Geometry check sheet. Reference: the model listing, model coordinates, mm. Face numbers are marked on the shaded views. A direction names the side the tool comes from. Coordinates: 2 decimals unless noted, no trailing zeros. Loops run counter-clockwise (first coordinate to the right, second up) from the corner with the lowest first, then second, coordinate; pieces in that order, holes last. Notation, with made-up numbers: (-7.5, -34.5) - (49.5, -34.5) arc R23 ccw to (49.5, -16.5) - close; hole circle Ø8 at (-13, 4.5). An arc over 180 degrees is marked (long way). One line per item, written item: value.
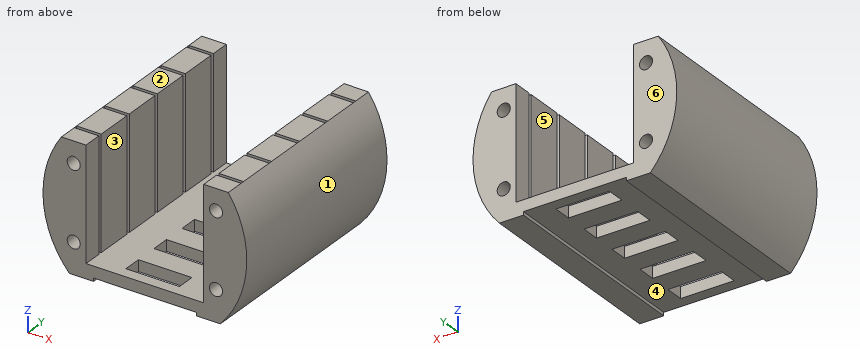
from build123d import *

# Parameters (mm, degrees)
BOSS_EXTRUDE2_DEPTH = 100
SKETCH2_W           = 26
SKETCH2_H           = 9
CUT_EXTRUDE1_DEPTH  = 10
SKETCH3_W           = 81.1
SKETCH3_H           = 1.7
CUT_EXTRUDE2_DEPTH  = 54.585490237
LPATTERN1_COUNT     = 5
LPATTERN1_PITCH     = 20
CUT_EXTRUDE3_START  = -100
SKETCH5_R           = 3.175
CUT_EXTRUDE3_DEPTH  = 100


with BuildPart() as part:
    # Sketch1 → Boss-Extrude2 (new body)
    with BuildSketch(Plane(origin=(0, 0, 0), x_dir=(1, 0, 0), z_dir=(0, 1, 0))):
        with BuildLine():
            Line((-40.55, -28.441490819), (-28.616848255, -28.441490819))
            Line((-28.616848255, -28.441490819), (-28.616848255, 26.143999418))
            Line((-28.616848255, 26.143999418), (28.616848255, 26.143999418))
            Line((28.616848255, 26.143999418), (28.616848255, -28.441490819))
            Line((28.616848255, -28.441490819), (40.55, -28.441490819))
            ThreePointArc((40.55, -28.441490819), (49.434601237, 3.072637396), (36.715901224, 33.243999418))
            Line((36.715901224, 33.243999418), (25, 33.243999418))
            Line((25, 33.243999418), (25, 31.643999418))
            Line((25, 31.643999418), (-25, 31.643999418))
            Line((-25, 31.643999418), (-25, 33.243999418))
            Line((-25, 33.243999418), (-36.715901224, 33.243999418))
            ThreePointArc((-36.715901224, 33.243999418), (-49.434601237, 3.072637396), (-40.55, -28.441490819))
        make_face()
    extrude(amount=BOSS_EXTRUDE2_DEPTH)

    # Sketch2 → Cut-Extrude1 (cut)
    with BuildSketch(Plane.XY.offset(-26.143999418)):
        with Locations((0, 10)):
            Rectangle(SKETCH2_W, SKETCH2_H)
    cut_extrude1 = extrude(amount=-CUT_EXTRUDE1_DEPTH, mode=Mode.SUBTRACT)

    # Sketch3 → Cut-Extrude2 (cut)
    with BuildSketch(Plane.XY.offset(28.441490819)):
        with Locations((0, 10)):
            Rectangle(SKETCH3_W, SKETCH3_H)
    cut_extrude2 = extrude(amount=-CUT_EXTRUDE2_DEPTH, mode=Mode.SUBTRACT)

    # LPattern1: Cut-Extrude1, Cut-Extrude2 ×5
    with Locations(*[(0, i * LPATTERN1_PITCH, 0) for i in range(1, LPATTERN1_COUNT)]):
        add(cut_extrude1, mode=Mode.SUBTRACT)
        add(cut_extrude2, mode=Mode.SUBTRACT)

    # Sketch5 → Cut-Extrude3 (cut)
    with BuildSketch(Plane(origin=(0, 100, 0), x_dir=(1, 0, 0), z_dir=(0, 1, 0)).offset(CUT_EXTRUDE3_START)):
        with Locations(Location((-34.583424127, -18.113346959, 0), (0, 0, 90))):
            Circle(SKETCH5_R)
        with Locations(Location((-34.583424127, 18.113346959, 0), (0, 0, 90))):
            Circle(SKETCH5_R)
        with Locations(Location((34.583424127, 18.113346959, 0), (0, 0, 90))):
            Circle(SKETCH5_R)
        with Locations(Location((34.583424127, -18.113346959, 0), (0, 0, 90))):
            Circle(SKETCH5_R)
    extrude(amount=CUT_EXTRUDE3_DEPTH, mode=Mode.SUBTRACT)


solid = part.part
(1) Cross-section at C-C on x = -16.5. Record the cut outline in (y, z), and give its area (3 significant figures).
Reply:
outline: (0, -31.64) - (100, -31.64) - (100, -26.14) - (0, -26.14) - close
area: 550 mm2
(2) Cross-section at A-A on y = 7. State how many separate pieces and enclosed holes the cut face has, and give its area (3 significant figures).
Reply:
separate pieces: 2
enclosed holes: 4
area: 2,210 mm2
(3) Release check for a two-part mould opening along X. For the marked faces 1, 2 and 3 record: pulls with the +X half, pulls with the -X half, needs draft (parallel to the pull), parting line crosses it, or undercut.
Reply:
face 1: pulls with the +X half
face 2: needs draft
face 3: undercut
(4) Go/stop test with flat-tipped pins: pin 1 Ø12 at (y, z) = (40.5, 14) entering from -X; pin 2 Ø8 at (y, z) = (90, -2.5) entering from -X; pin 3 Ø12 at (y, z) = (35, 8.5) entering from +X. Record where each tip stops, or that it passes through.
Reply:
pin 1: x = -48.88
pin 2: x = -49.53
pin 3: x = 49.47
(5) Material ranges on probe 1 along X at (y, z) = (10, -1.5); probe 2 along Z at (x, y) = (-35, 26); probe 3 along Z at (x, y) = (14.5, 62), recorded low to high. Write a range as from..to.
Reply:
probe 1: -49.51..-40.55, 40.55..49.51
probe 2: -33.24..-21.26, -14.97..14.97, 21.26..28.44
probe 3: -31.64..-26.14
(6) Access from +Z, -Z, +X, -X, +Y, -Y to the whole of each face (thin tool, end or side, straight path). Record for the marked faces 4, 5 and 6.
Reply:
face 4: -Z, +Y, -Y
face 5: +Z, +Y, -Y
face 6: +Z, -Z, +X, -X, +Y
